Could you check a few things on this model? Use its own coordinates, in mm. Round coordinates to 2 decimals unless told otherwise and drop trailing zeros. Write each loop counter-clockwise with the first axis right and the second up, starting at its lowest first coordinate (ties: lowest second). Pieces come first, ordered by that corner, then holes. Notation, with made-up numbers: (6, 20.5) -> (39, 20.5) arc R25 ccw to (39, 58.5) -> close; hole circle Ø1 at (-18, 12.5). An arc over 180 degrees is marked (long way). Return JSON: item names as keys, results as strings.
from build123d import *

# Parameters (mm, degrees)
SKETCH_1_R      = 4
SKETCH_1_R_2    = 2.5
SKETCH_1_R_3    = 1.45
EXTRUDE_1_DEPTH = 15
CHAMFER_1_SIZE  = 1.8
CHAMFER_2_SIZE  = 2.7


with BuildPart() as part:
    # 草图1 → 凸台-拉伸1 (new body)
    with BuildSketch(Plane(origin=(0, 0, 0), x_dir=(1, 0, 0), z_dir=(0, 1, 0))):
        with BuildLine():
            Line((-0.574418605, 18.991314943), (214.229069767, 25.488343739))
            ThreePointArc((214.229069767, 25.488343739), (240.5, 0), (214.229069767, -25.488343739))
            Line((214.229069767, -25.488343739), (-0.574418605, -18.991314943))
            ThreePointArc((-0.574418605, -18.991314943), (-19, 0), (-0.574418605, 18.991314943))
        make_face()
        with Locations(Location((0, 0, 0), (0, 0, 270))):
            Circle(SKETCH_1_R, mode=Mode.SUBTRACT)
        with Locations(Location((209.5, 9.526279442, 0), (0, 0, 270))):
            Circle(SKETCH_1_R_2, mode=Mode.SUBTRACT)
        with Locations(Location((220.5, 9.526279442, 0), (0, 0, 270))):
            Circle(SKETCH_1_R_2, mode=Mode.SUBTRACT)
        with Locations(Location((226, 0, 0), (0, 0, 270))):
            Circle(SKETCH_1_R_2, mode=Mode.SUBTRACT)
        with Locations(Location((220.5, -9.526279442, 0), (0, 0, 270))):
            Circle(SKETCH_1_R_2, mode=Mode.SUBTRACT)
        with Locations(Location((209.5, -9.526279442, 0), (0, 0, 270))):
            Circle(SKETCH_1_R_2, mode=Mode.SUBTRACT)
        with Locations(Location((204, 0, 0), (0, 0, 270))):
            Circle(SKETCH_1_R_2, mode=Mode.SUBTRACT)
        with Locations(Location((-5.656854249, 5.656854249, 0), (0, 0, 270))):
            Circle(SKETCH_1_R_3, mode=Mode.SUBTRACT)
        with Locations(Location((5.656854249, 5.656854249, 0), (0, 0, 270))):
            Circle(SKETCH_1_R_3, mode=Mode.SUBTRACT)
        with Locations(Location((5.656854249, -5.656854249, 0), (0, 0, 270))):
            Circle(SKETCH_1_R_3, mode=Mode.SUBTRACT)
        with Locations(Location((-5.656854249, -5.656854249, 0), (0, 0, 270))):
            Circle(SKETCH_1_R_3, mode=Mode.SUBTRACT)
    extrude(amount=EXTRUDE_1_DEPTH)

    # 倒角1
    chamfer_1_edges = [part.edges().sort_by_distance(p)[0] for p in [
        (5.656854249, 0, -7.106854249),
        (-5.656854249, 0, -7.106854249),
        (5.656854249, 0, 4.206854249),
        (-5.656854249, 0, 4.206854249),
    ]]
    chamfer(chamfer_1_edges, length=CHAMFER_1_SIZE)

    # 倒角2
    chamfer_2_edges = [part.edges().sort_by_distance(p)[0] for p in [
        (209.5, 0, -12.026279442),
        (226, 0, -2.5),
        (209.5, 0, 7.026279442),
    ]]
    chamfer(chamfer_2_edges, length=CHAMFER_2_SIZE)


solid = part.part
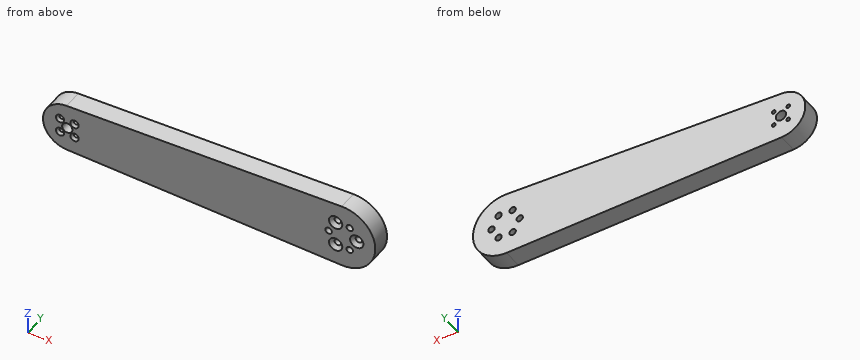
1) I want a section at C-C, the plane x = 226. Please give me the cut outline in (y, z).
Return value:
{"outline": "(0, -23.01) -> (15, -23.01) -> (15, -2.5) -> (2.7, -2.5) -> (0, -5.2) -> close; (0, 5.2) -> (2.7, 2.5) -> (15, 2.5) -> (15, 23.01) -> (0, 23.01) -> close"}
2) If I drill on probe 1 along X at (y, z) = (10, 0); probe 2 along Z at (x, y) = (209.5, 7.25); probe 3 along Z at (x, y) = (221, 8.25), over which ranges is the centre line in solid material (lowest first)? Write a range as [from, to].
Return value:
{"probe 1": "[-19, -4], [4, 201.5], [206.5, 223.5], [228.5, 240.5]", "probe 2": "[-25.35, -12.03], [-7.03, 7.03], [12.03, 25.35]", "probe 3": "[-24.78, -11.98], [-7.08, 7.08], [11.98, 24.78]"}
3) I want a section at B-B, the plane y = 9. Count the separate pieces of the cut face and the enclosed holes in it, and give its area (3 significant figures).
Return value:
{"separate pieces": "1", "enclosed holes": "11", "area": "11,000 mm²"}
4) I want a section at D-D, the plane x = 90. Please give me the cut outline in (y, z), and give its area (3 significant figures).
Return value:
{"outline": "(0, -21.73) -> (15, -21.73) -> (15, 21.73) -> (0, 21.73) -> close", "area": "652 mm²"}
5) Will these pins go through, and if not, where does the flat tip stop? pin 1 Ø4 at (x, y) = (66.5, 11.5) entering from +Z; pin 2 Ø6.5 at (x, z) = (226, 0) entering from +Y; pin 3 Ø5 at (y, z) = (3.5, -14.5) entering from +X; pin 4 Ø2 at (x, y) = (210, 4) entering from -Z.
Return value:
{"pin 1": "z = 21.08", "pin 2": "y = 15", "pin 3": "x = 237.5", "pin 4": "z = -25.39"}
6) I want a section at A-A, the plane z = 0. Please give me the cut outline in (x, y), and give its area (3 significant figures).
Return value:
{"outline": "(-19, 0) -> (-4, 0) -> (-4, 15) -> (-19, 15) -> close; (4, 0) -> (201.5, 0) -> (201.5, 15) -> (4, 15) -> close; (206.5, 0) -> (220.8, 0) -> (223.5, 2.7) -> (223.5, 15) -> (206.5, 15) -> close; (228.5, 2.7) -> (231.2, 0) -> (240.5, 0) -> (240.5, 15) -> (228.5, 15) -> close", "area": "3,620 mm²"}
